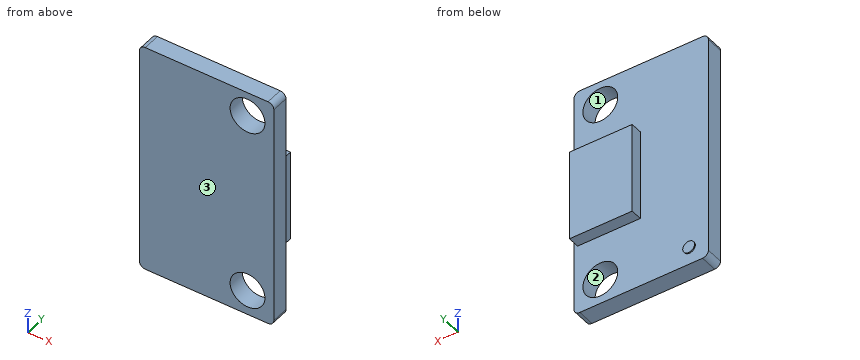
from build123d import *

# Parameters (mm, degrees)
SKETCH1_W           = 11.566360694
SKETCH1_H           = 20.211316514
BOSS_EXTRUDE1_DEPTH = 1.5
SKETCH1_4_W         = 5.4
SKETCH1_4_H         = 7.9
BOSS_EXTRUDE2_DEPTH = 1
SKETCH1_5_R         = 0.51
BOSS_EXTRUDE3_DEPTH = 0.1
SKETCH2_R           = 1.5
CUT_EXTRUDE1_DEPTH  = 2.1
FILLET1_R           = 0.5


with BuildPart() as part:
    # Sketch1 → Boss-Extrude1 (new body)
    with BuildSketch(Plane(origin=(0, 0, 0), x_dir=(1, 0, 0), z_dir=(0, 1, 0))):
        with Locations((-2.777214228, -0.021219212)):
            Rectangle(SKETCH1_W, SKETCH1_H)
    extrude(amount=-BOSS_EXTRUDE1_DEPTH)

    # Sketch1_4 → Boss-Extrude2 (add)
    with BuildSketch(Plane(origin=(0, 0, 0), x_dir=(1, 0, 0), z_dir=(0, 1, 0))):
        Rectangle(SKETCH1_4_W, SKETCH1_4_H)
    extrude(amount=BOSS_EXTRUDE2_DEPTH)

    # Sketch1_5 → Boss-Extrude3 (add)
    with BuildSketch(Plane(origin=(0, 0, 0), x_dir=(1, 0, 0), z_dir=(0, 1, 0))):
        with Locations(Location((-6.930111953, 8.586389213, 0), (0, 0, 270))):
            Circle(SKETCH1_5_R)
    extrude(amount=BOSS_EXTRUDE3_DEPTH)

    # Sketch2 → Cut-Extrude1 (cut)
    with BuildSketch(Plane(origin=(0, 0, 0), x_dir=(1, 0, 0), z_dir=(0, 1, 0))):
        with Locations(Location((0.741742268, 7.899498536, 0), (0, 0, 270))):
            Circle(SKETCH2_R)
        with Locations(Location((0.741742268, -8.032859578, 0), (0, 0, 270))):
            Circle(SKETCH2_R)
    extrude(amount=-CUT_EXTRUDE1_DEPTH, mode=Mode.SUBTRACT)

    # Fillet1
    fillet1_edges = [part.edges().sort_by_distance(p)[0] for p in [
        (-8.560394575, -0.75, -10.084439045),
        (3.005966119, -0.75, -10.084439045),
        (3.005966119, -0.75, 10.126877469),
        (-8.560394575, -0.75, 10.126877469),
    ]]
    fillet(fillet1_edges, radius=FILLET1_R)


solid = part.part
Work out the finished part from the listing and answer in its coordinate system (mm). Face numbers are marked on the shaded views. Give positions to 0.01 mm unless a question says otherwise; leave off trailing zeros. Loops run counter-clockwise (first coordinate to the right, second up) from the corner with the lowest first, then second, coordinate; pieces in that order, holes last. Notation, with made-up numbers: (36.25, 40) - (81.25, 40) arc R13 cw to (81.25, 53) - close; hole circle Ø6 at (79, -30.5). An arc over 180 degrees is marked (long way). Answer in a Markdown table with one row per item. Add a question column.
Q1. Determine the mould class of the marked faces 1, 2 and 3 for opening direction X: released by +X, released by -X, zero draft, split by the parting line, or undercut.
Q2. The part is cut by section C-C (x = 0.5). Determine the outline of the cut face in (y, z), and give its area (3 significant figures).
Q3. The part is cut by section A-A (z = 7.75). Determine the outline of the cut face in (x, y).
Q4. Consider line 1 along Z through (x, y) = (-0.5, -1.2); line 2 along Z through (x, y) = (0, -0.05); line 3 along Y through (x, z) = (-7.25, 7.5). Determine where each line is inside the solid, lowest interval first.
Q5. The part is cut by section D-D (z = -2.75). Determine the outline of the cut face in (x, y).
Q6. Each of these flat-tipped pins is pushed along its axis until it touches: P1, Ø0.5, axis at x = 1, y = 0.5, coming from the +Z side; P2, Ø0.8, axis at x = 0, y = 0.5, coming from the -Z side; P3, Ø0.5, axis at x = -7, z = -8.5, coming from the +Y side. Where does it stop, or does it pass through?
Q7. The part is cut by section B-B (y = -1.1). Determine the outline of the cut face in (x, z), and give its area (3 significant figures).
Solution:
| question | item | result |
|---|---|---|
| 1 | face 1 | undercut |
| 1 | face 2 | undercut |
| 1 | face 3 | zero draft |
| 2 | outline | (-1.5, -10.08) - (0, -10.08) - (0, -9.38) - (-1.5, -9.38) - close; (-1.5, -6.42) - (0, -6.42) - (0, -3.95) - (1, -3.95) - (1, 3.95) - (0, 3.95) - (0, 6.55) - (-1.5, 6.55) - close; (-1.5, 9.51) - (0, 9.51) - (0, 10.13) - (-1.5, 10.13) - close |
| 2 | area | 29.3 mm² |
| 3 | outline | (-8.56, -1.5) - (-0.73, -1.5) - (-0.73, 0) - (-8.56, 0) - close; (2.21, -1.5) - (3.01, -1.5) - (3.01, 0) - (2.21, 0) - close |
| 4 | line 1 | z = -10.08 to -8.74, -7.06 to 7.19, 8.87 to 10.13 |
| 4 | line 2 | z = -10.08 to -9.2, -6.6 to 6.73, 9.34 to 10.13 |
| 4 | line 3 | y = -1.5 to 0 |
| 5 | outline | (-8.56, -1.5) - (3.01, -1.5) - (3.01, 0) - (2.7, 0) - (2.7, 1) - (-2.7, 1) - (-2.7, 0) - (-8.56, 0) - close |
| 6 | P1 | stops at z = 3.95 |
| 6 | P2 | stops at z = -3.95 |
| 6 | P3 | stops at y = 0.1 |
| 7 | outline | (-8.56, -9.58) arc R0.5 ccw to (-8.06, -10.08) - (2.51, -10.08) arc R0.5 ccw to (3.01, -9.58) - (3.01, 9.63) arc R0.5 ccw to (2.51, 10.13) - (-8.06, 10.13) arc R0.5 ccw to (-8.56, 9.63) - close; hole circle Ø3 at (0.74, -7.9); hole circle Ø3 at (0.74, 8.03) |
| 7 | area | 219 mm² |
